Design review of the part built by this model. Coordinates are the model's own, in mm. A direction names the side the tool comes from. Give positions to 0.01 mm unless a question says otherwise; leave off trailing zeros. Order: outer loops, then holes, each group sorted by start corner. A loop starts at its lowest first (then second) coordinate and runs counter-clockwise, first axis right, second up. Notation, with made-up numbers: (41, 27.5) -> (72, 27.5) arc R13 cw to (72, 40.5) -> close; hole circle Ø1 at (66.25, -8.75). An arc over 180 degrees is marked (long way). Return JSON: item names as keys, results as strings.
```python
from build123d import *

# Parameters (mm, degrees)
F0_W     = 76.2
F0_H     = 50.8
F1_DEPTH = 101.6
F3_W     = 71.12
F3_H     = 96.52
F4_DEPTH = 44.45
F2_R     = 11.43
F5_DEPTH = 5.08
F2_W     = 20.32
F2_H     = 31.75
F6_DEPTH = 1.27
F7_W     = 12.7
F7_H     = 12.7
F7_W_2   = 10.16
F7_H_2   = 10.16
F8_DEPTH = 50.8
F9_DEPTH = 50.801


with BuildPart() as f1:
    # F0 (on Top) → F1 (new body)
    with BuildSketch(Plane.XY):
        Polygon((38.1, 84.401042), (0, 50.8), (76.2, 50.8), align=None)
        with Locations((38.1, 25.4)):
            Rectangle(F0_W, F0_H)
    extrude(amount=F1_DEPTH)

    # F3 (on face) → F4 (cut)
    with BuildSketch(Plane.XZ):
        with Locations((38.1, 50.8)):
            Rectangle(F3_W, F3_H)
    extrude(amount=-F4_DEPTH, mode=Mode.SUBTRACT)

    # F2 (on face) → F5 (cut)
    with BuildSketch(Plane.XY.offset(101.6)):
        with Locations((38.1, 57.15)):
            Circle(F2_R)
    extrude(amount=-F5_DEPTH, mode=Mode.SUBTRACT)

    # F2 (on face) → F6 (cut)
    with BuildSketch(Plane.XY.offset(101.6)):
        with Locations((38.1, 15.875)):
            Rectangle(F2_W, F2_H)
        with Locations((38.1, 57.15)):
            Circle(F2_R)
    extrude(amount=-F6_DEPTH, mode=Mode.SUBTRACT)

    # F7 (on face) → F8 (join)
    with BuildSketch(Plane.XZ.offset(-44.45)):
        with Locations((44.45, 19.05)):
            Rectangle(F7_W, F7_H)
        with Locations((44.45, 19.05)):
            Rectangle(F7_W_2, F7_H_2, mode=Mode.SUBTRACT)
    extrude(amount=-F8_DEPTH)

    # F7 (on face) → F9 (cut, through all)
    with BuildSketch(Plane.XZ.offset(-44.45)):
        with Locations((44.45, 19.05)):
            Rectangle(F7_W_2, F7_H_2)
    extrude(amount=-F9_DEPTH, mode=Mode.SUBTRACT)


solid = f1.part
```
Item 1: Mouldability with a two-part tool opening along Y and no side actions: class faces 4 (the face through (38, 57, 96.52)), 5 (the face through (44, 87, 12.7)), 6 (the face through (44, 95.25, 13)) as released by +Y, released by -Y, zero draft, split by the parting line, or undercut.
Result set:
{"face 4": "undercut", "face 5": "zero draft", "face 6": "released by +Y"}
Item 2: Add section C-C (x = 12). Give the boundary of the cut face in (y, z).
Result set:
{"outline": "(0, 0) -> (61.38, 0) -> (61.38, 101.6) -> (0, 101.6) -> (0, 99.06) -> (44.45, 99.06) -> (44.45, 2.54) -> (0, 2.54) -> close"}
Item 3: Add section D-D (y = 57.15). Give the boundary of the cut face in (x, z), plus the area to 3 significant figures.
Result set:
{"outline": "(7.2, 0) -> (69, 0) -> (69, 101.6) -> (49.53, 101.6) -> (49.53, 96.52) -> (26.67, 96.52) -> (26.67, 101.6) -> (7.2, 101.6) -> close; hole (39.37, 13.97) -> (49.53, 13.97) -> (49.53, 24.13) -> (39.37, 24.13) -> close", "area": "6,060 mm^2"}
Item 4: Machinability: for faces 1 (the face through (38.1, 90, 19)), 2 (the face through (50.8, 84, 19)), 3 (the face through (39.37, 69, 19)), which of the approach directions +Z, -Z, +X, -X, +Y, -Y give a long, thin tool a straight path to every point of the face, cutting with its end or side? Answer none if there is none.
Result set:
{"face 1": "+Z, -Z, -X, +Y", "face 2": "+Z, -Z, +X, +Y", "face 3": "+Y, -Y"}
Item 5: Add section A-A (y = 28). Give the boundary of the cut face in (x, z).
Result set:
{"outline": "(0, 0) -> (76.2, 0) -> (76.2, 101.6) -> (48.26, 101.6) -> (48.26, 100.33) -> (27.94, 100.33) -> (27.94, 101.6) -> (0, 101.6) -> close; hole (2.54, 2.54) -> (73.66, 2.54) -> (73.66, 99.06) -> (2.54, 99.06) -> close"}
Item 6: Add section B-B (z = 31). Give the boundary of the cut face in (x, y), plus the area to 3 significant figures.
Result set:
{"outline": "(0, 0) -> (2.54, 0) -> (2.54, 44.45) -> (73.66, 44.45) -> (73.66, 0) -> (76.2, 0) -> (76.2, 50.8) -> (38.1, 84.4) -> (0, 50.8) -> close", "area": "1,990 mm^2"}
Item 7: Wall thickness on L1, parallel to Z at x = 61.5, y = 36.5; L2, parallel to X at y = 18, z = 86.5; L3, parallel to Y at x = 38.1, z = 99.7: over which ranges is each line inside the solid? List them lowest first. Write a range as [from, to].
Result set:
{"L1": "z = [0, 2.54], [99.06, 101.6]", "L2": "x = [0, 2.54], [73.66, 76.2]", "L3": "y = [0, 45.72], [68.58, 84.4]"}
Item 8: For pin 1 (6 mm diameter, centred on x = 36.5, y = 13, fed in from +Z); pin 2 (1 mm diameter, centred on x = 42, z = 101, fed in from -Y); pin 3 (3.5 mm diameter, centred on y = 89.5, z = 20.5, fed in from -X), all flat-tipped, find the tip position at first contact; note any pin that passes through.
Result set:
{"pin 1": "stops at z = 100.33", "pin 2": "stops at y = 31.75", "pin 3": "stops at x = 38.1"}
